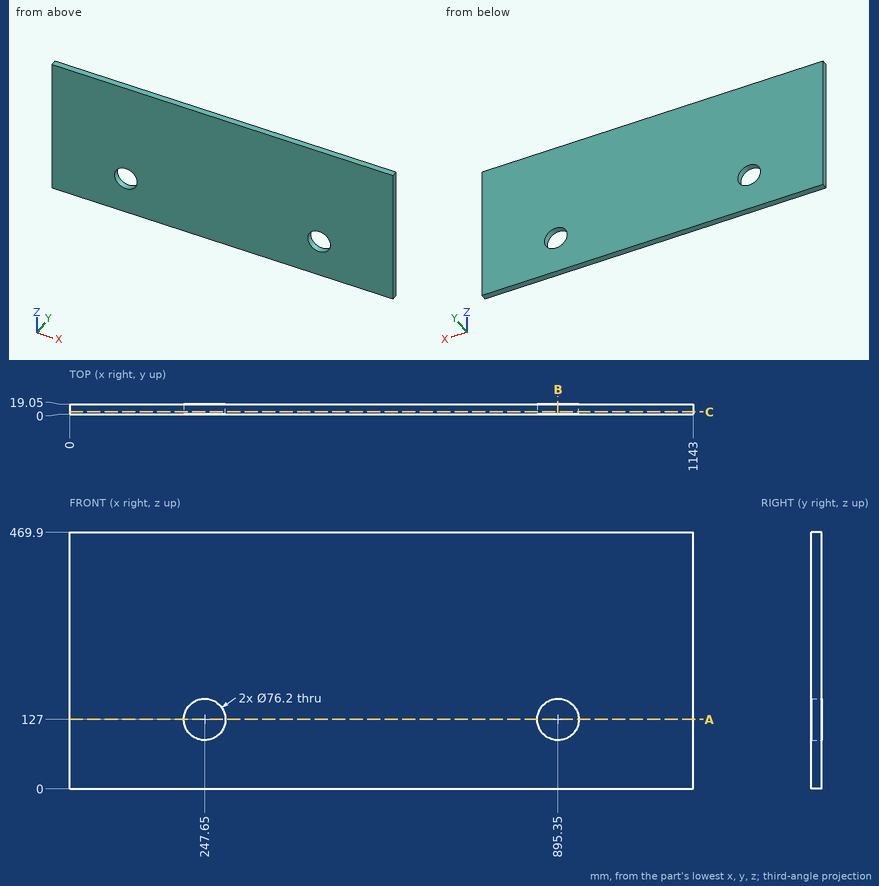
Part print with two shaded views. Sizes in mm from the minimum x, y, z corner. Give positions to 0.01 mm unless a question says otherwise; leave off trailing zeros. Write each loop counter-clockwise with the first axis right and the second up, starting at its lowest first coordinate (ties: lowest second). Pieces come first, ordered by that corner, then holes.
1) Cut at C-C on y = 4.5. Write the cut outline in (x, z).
Resolved:
outline: (0, 0) - (1143, 0) - (1143, 469.9) - (0, 469.9) - close; hole circle Ø76.2 at (247.65, 127); hole circle Ø76.2 at (895.35, 127)
2) Cut at A-A on z = 127. Write the cut outline in (x, y), then the cut area to 3 significant figures.
Resolved:
outline: (0, 0) - (209.55, 0) - (209.55, 19.05) - (0, 19.05) - close; (285.75, 0) - (857.25, 0) - (857.25, 19.05) - (285.75, 19.05) - close; (933.45, 0) - (1143, 0) - (1143, 19.05) - (933.45, 19.05) - close
area: 18,900 mm2
3) Cut at B-B on x = 895.35. Write the cut outline in (y, z).
Resolved:
outline: (0, 0) - (19.05, 0) - (19.05, 88.9) - (0, 88.9) - close; (0, 165.1) - (19.05, 165.1) - (19.05, 469.9) - (0, 469.9) - close
4) Probe L1, parallel to Z at x = 895.35, y = 9.75; L2, parallel to Z at x = 260.5, y = 9.5. List the from-to ranges inside material, lowest first.
Resolved:
L1: z = 0 to 88.9, 165.1 to 469.9
L2: z = 0 to 91.13, 162.87 to 469.9
